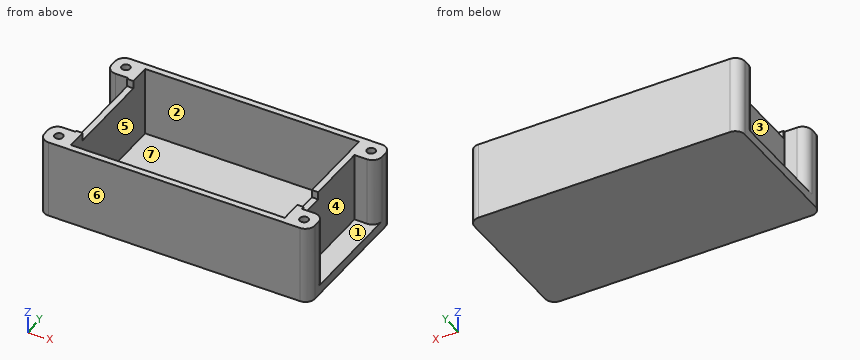
from build123d import *

# Parameters (mm, degrees)
F0_W     = 86
F0_H     = 45
F1_DEPTH = 3
F2_R     = 1.35
F2_W     = 68
F2_H     = 41
F3_DEPTH = 22
F4_R     = 3
F5_W     = 2
F5_H     = 28
F5_H_2   = 8
F6_DEPTH = 2.5


# Not quite as in the source:
# - a feature names something its author has since deleted; it is built from what else it names


with BuildPart() as f1:
    # F0 (on Top) → F1 (new body)
    with BuildSketch(Plane.XY):
        Rectangle(F0_W, F0_H)
    extrude(amount=F1_DEPTH)

    # F2 (on face) → F3 (join)
    with BuildSketch(Plane.XY.offset(3)):
        Polygon((43, 22.5), (-43, 22.5), (-43, 14.5), (-36, 14.5), (-36, -14.5), (-43, -14.5), (-43, -22.5), (43, -22.5), (43, -14.5), (36, -14.5), (36, 14.5), (43, 14.5), align=None)
        with Locations((-39, -18.5)):
            Circle(F2_R, mode=Mode.SUBTRACT)
        with Locations((39, -18.5)):
            Circle(F2_R, mode=Mode.SUBTRACT)
        with Locations((-39, 18.5)):
            Circle(F2_R, mode=Mode.SUBTRACT)
        Rectangle(F2_W, F2_H, mode=Mode.SUBTRACT)
        with Locations((39, 18.5)):
            Circle(F2_R, mode=Mode.SUBTRACT)
    extrude(amount=F3_DEPTH)

    # F4
    f4_edges = [f1.edges().sort_by_distance(p)[0] for p in [
        (-43, -22.5, 12.5),
        (-43, 14.5, 14),
        (-43, 22.5, 12.5),
        (-43, -14.5, 14),
        (43, -22.5, 12.5),
        (43, -14.5, 14),
        (43, 14.5, 14),
        (43, 22.5, 12.5),
    ]]
    fillet(f4_edges, radius=F4_R)

    # F5 (on face) → F6 (cut)
    with BuildSketch(Plane.XY.offset(25)):
        with Locations((-35, 0)):
            Rectangle(F5_W, F5_H)
        with Locations((35, -9.5)):
            Rectangle(F5_W, F5_H_2)
    extrude(amount=-F6_DEPTH, mode=Mode.SUBTRACT)


solid = f1.part
For this review, take the finished solid that the model builds, in its own axes (mm). Face numbers are marked on the shaded views. A direction names the side the tool comes from. Round coordinates to 2 decimals unless told otherwise and drop trailing zeros. Loops run counter-clockwise (first coordinate to the right, second up) from the corner with the lowest first, then second, coordinate; pieces in that order, holes last. Notation, with made-up numbers: (49.25, -18) - (69.25, -18) arc R21 ccw to (69.25, 3) - close; hole circle Ø9 at (56.25, -15). An arc over 180 degrees is marked (long way). One line per item, written item: value. Start each with the question number.
Item 1: For L1, parallel to Y at x = 39, z = 14.75; L2, parallel to X at y = -2.5, z = 6.75; L3, parallel to Y at x = -4, z = 14.5, list the stretches that pass through material, from the lowest coordinate up.
Item 2: Take a section at C-C (x = 13.5). Give the boundary of the cut face in (y, z).
Item 3: Take a section at D-D (y = -18.5). Give the boundary of the cut face in (x, z), plus the area to 3 significant figures.
Item 4: Clearance check with flat-ended pins moving along their axes: pin 1 Ø1 at (y, z) = (7.5, 7.5) entering from -X; pin 2 Ø2 at (x, y) = (-35, 0.5) entering from +Z; pin 3 Ø6 at (x, y) = (26, -5) entering from +Z. State where each tip first meets the part, or that it passes through.
Item 5: For the marked faces 1, 2 and 3, list the 3-axis set-ups (+Z, -Z, +X, -X, +Y, -Y) from which the entire face can be reached by the end or side of a thin tool; tool diameter is ignored.
Item 6: Take a section at A-A (z = 10.5). Give the boundary of the cut face in (x, y).
Item 7: Take a section at B-B (y = -4.5). Give the boundary of the cut face in (x, z).
Item 8: The part is to be moulded in two halves that separate along X. For the marked faces 4, 5, 6 and 7, say which applies: +X half, -X half, draft (parallel to the pull), parting line (faces both ways), or undercut.
Answer below:
1. L1: y = -22.5 to -19.85, -17.15 to -14.5, 14.5 to 17.15, 19.85 to 22.5
1. L2: x = -36 to -34, 34 to 36
1. L3: y = -22.5 to -20.5, 20.5 to 22.5
2. outline: (-22.5, 0) - (22.5, 0) - (22.5, 25) - (20.5, 25) - (20.5, 3) - (-20.5, 3) - (-20.5, 25) - (-22.5, 25) - close
3. outline: (-43, 0) - (43, 0) - (43, 25) - (40.35, 25) - (40.35, 3) - (37.65, 3) - (37.65, 25) - (34, 25) - (34, 3) - (-34, 3) - (-34, 25) - (-37.65, 25) - (-37.65, 3) - (-40.35, 3) - (-40.35, 25) - (-43, 25) - close
3. area: 535 mm2
4. pin 1: stops at x = -36
4. pin 2: stops at z = 22.5
4. pin 3: stops at z = 3
5. face 1: +Z, +X
5. face 2: +Z
5. face 3: +Z, -X
6. outline: (-43, -19.5) arc R3 ccw to (-40, -22.5) - (40, -22.5) arc R3 ccw to (43, -19.5) - (43, -17.5) arc R3 ccw to (40, -14.5) - (36, -14.5) - (36, 14.5) - (40, 14.5) arc R3 ccw to (43, 17.5) - (43, 19.5) arc R3 ccw to (40, 22.5) - (-40, 22.5) arc R3 ccw to (-43, 19.5) - (-43, 17.5) arc R3 ccw to (-40, 14.5) - (-36, 14.5) - (-36, -14.5) - (-40, -14.5) arc R3 ccw to (-43, -17.5) - close; hole circle Ø2.7 at (-39, -18.5); hole circle Ø2.7 at (-39, 18.5); hole (-34, -20.5) - (34, -20.5) - (34, 20.5) - (-34, 20.5) - close; hole circle Ø2.7 at (39, -18.5); hole circle Ø2.7 at (39, 18.5)
7. outline: (-43, 0) - (43, 0) - (43, 3) - (36, 3) - (36, 25) - (34, 25) - (34, 3) - (-34, 3) - (-34, 22.5) - (-36, 22.5) - (-36, 3) - (-43, 3) - close
8. face 4: +X half
8. face 5: undercut
8. face 6: draft
8. face 7: undercut
